Here's the drawing with two shaded views (mm, measured from the low corner). I have some questions. A direction names the side the tool comes from. Give positions to 0.01 mm unless a question says otherwise; leave off trailing zeros. Write each loop counter-clockwise with the first axis right and the second up, starting at its lowest first coordinate (ties: lowest second). Pieces come first, ordered by that corner, then holes.
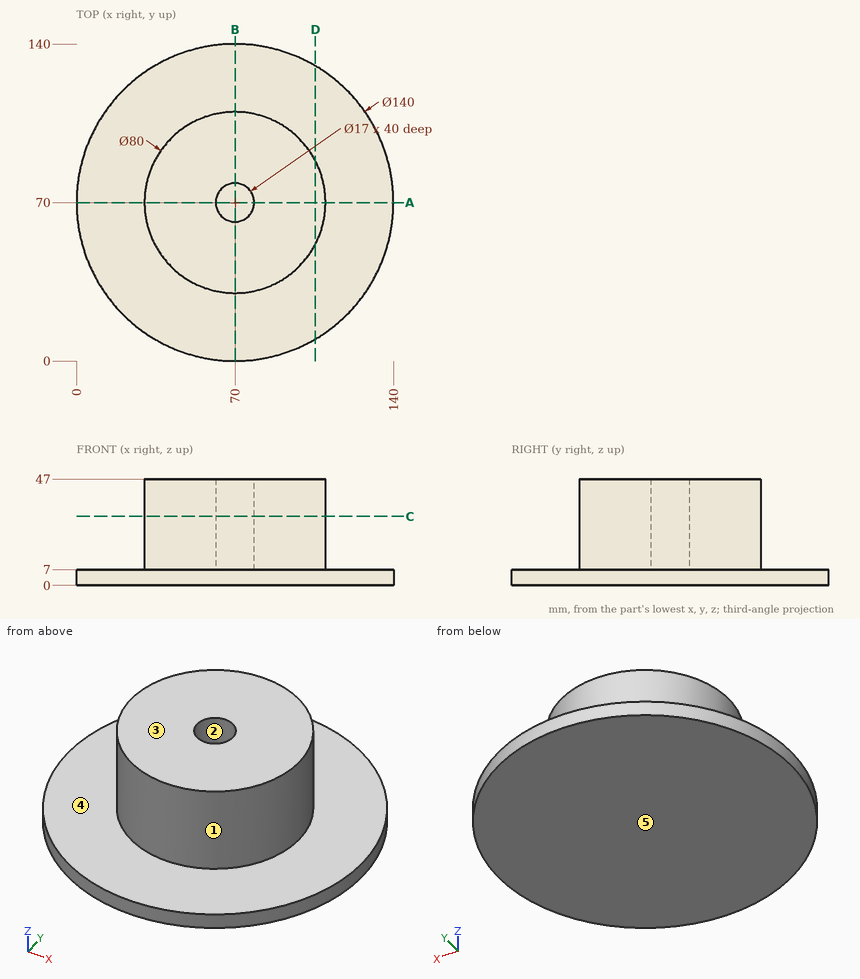
(1) Will these pins go through, and if not, where does the flat tip stop? P1, Ø6, axis at x = 19, y = 57.5, coming from the -Z side; P2, Ø1, axis at y = 47, z = 8, coming from the -X side; P3, Ø6, axis at y = 65, z = 19.5, coming from the +X side; P4, Ø4, axis at y = 102, z = 15, coming from the +X side.
Returned:
P1: stops at z = 0
P2: stops at x = 36.93
P3: stops at x = 109.95
P4: stops at x = 96.46
(2) For the marked faces 4 and 5, which set-ups out of +Z, -Z, +X, -X, +Y, -Y let a thin tool reach every point of the face, with its end or its side?
Returned:
face 4: +Z
face 5: -Z, +X, -X, +Y, -Y
(3) If we mould it in two halves opening along X, with no side actions, what happens to the marked faces 1, 2 and 3? For each: +X half, -X half, draft (parallel to the pull), parting line (faces both ways), or undercut.
Returned:
face 1: parting line
face 2: undercut
face 3: draft
(4) Imagine slicing it at D-D, the plane x = 105.5. Write out the boundary of the cut face in (y, z), plus the area to 3 significant figures.
Returned:
outline: (9.67, 0) - (130.33, 0) - (130.33, 7) - (88.43, 7) - (88.43, 47) - (51.57, 47) - (51.57, 7) - (9.67, 7) - close
area: 2,320 mm2
(5) Imagine slicing it at C-C, the plane z = 30.5. Write out the boundary of the cut face in (x, y).
Returned:
outline: circle Ø80 at (70, 70); hole circle Ø17 at (70, 70)
(6) Imagine slicing it at A-A, the plane y = 70. Write out the boundary of the cut face in (x, z).
Returned:
outline: (0, 0) - (140, 0) - (140, 7) - (110, 7) - (110, 47) - (78.5, 47) - (78.5, 7) - (61.5, 7) - (61.5, 47) - (30, 47) - (30, 7) - (0, 7) - close
(7) If I drill on L1, parallel to Y at x = 70, z = 16; L2, parallel to Z at x = 115.5, y = 46; L3, parallel to Y at x = 40, z = 29.5, over which ranges is the centre line in solid material (lowest first)?
Returned:
L1: y = 30 to 61.5, 78.5 to 110
L2: z = 0 to 7
L3: y = 43.54 to 96.46
